Drawing for the job (mm, zero at the part's lowest x, y, z). A direction names the side the tool comes from. Give positions to 0.01 mm unless a question says otherwise; leave off trailing zeros. Loops run counter-clockwise (first coordinate to the right, second up) from the corner with the lowest first, then second, coordinate; pieces in that order, holes last. Notation, with made-up numbers: (56.25, 54) - (62.25, 54) arc R24 cw to (62.25, 69) - close; hole circle Ø7 at (-23.75, 55.5). An arc over 180 degrees is marked (long way). Return JSON: item names as keys, results as strings. Group by question number.
1) Drill centre lines: probe 1 along X at (y, z) = (75, 12.5); probe 2 along Z at (x, y) = (63.5, 78.5); probe 3 along X at (y, z) = (26.5, 34). Where is each one in solid material? Low to high. Write a range as from..to.
2) Mould opens along Z. For the marked faces 3, 4, 5 and 6 say: released by +Z, released by -Z, zero draft, split by the parting line, or undercut.
3) 3-axis set-ups, long thin cutter, end or side, ignore diameter. For the marked faces 1 and 2: which of +Z, -Z, +X, -X, +Y, -Y reach the whole face in a straight line?
4) Drop flat-ended pins along their axis: pin 1 (4 mm diameter, centred on x = 40, y = 16.5, fed in from +Z); pin 2 (1 mm diameter, centred on x = 49, z = 7.5, fed in from -Y). Give the stop position or say it passes through.
5) Slice it at D-D (z = 25.4). List the corners of the cut face in (x, y).
6) Slice it at B-B (y = 37). List the corners of the cut face in (x, z).
7) Slice it at A-A (x = 63.5). List the corners of the cut face in (y, z).
8) Slice it at C-C (z = 17). List the corners of the cut face in (x, y).
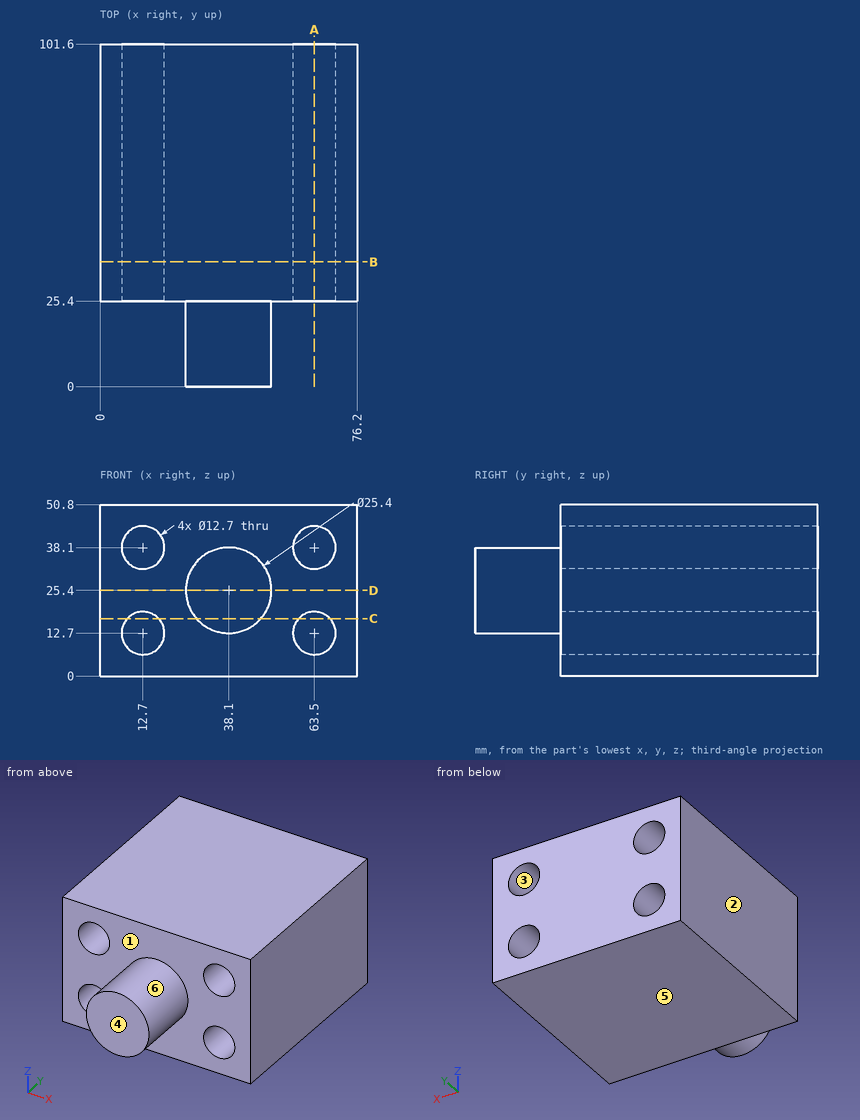
Results:
{
 "1": {"probe 1": "0..6.35, 19.05..57.15, 69.85..76.2", "probe 2": "0..6.35, 19.05..31.75, 44.45..50.8", "probe 3": "0..7.85, 17.55..58.65, 68.35..76.2"},
 "2": {"face 3": "undercut", "face 4": "zero draft", "face 5": "released by -Z", "face 6": "split by the parting line"},
 "3": {"face 1": "-Y", "face 2": "+Z, -Z, -X, +Y, -Y"},
 "4": {"pin 1": "z = 38.1", "pin 2": "y = 25.4"},
 "5": {"outline": "(0, 25.4) - (25.4, 25.4) - (25.4, 0) - (50.8, 0) - (50.8, 25.4) - (76.2, 25.4) - (76.2, 101.6) - (0, 101.6) - close"},
 "6": {"outline": "(0, 0) - (76.2, 0) - (76.2, 50.8) - (0, 50.8) - close; hole circle Ø12.7 at (12.7, 12.7); hole circle Ø12.7 at (12.7, 38.1); hole circle Ø12.7 at (63.5, 12.7); hole circle Ø12.7 at (63.5, 38.1)"},
 "7": {"outline": "(25.4, 0) - (101.6, 0) - (101.6, 6.35) - (25.4, 6.35) - close; (25.4, 19.05) - (101.6, 19.05) - (101.6, 31.75) - (25.4, 31.75) - close; (25.4, 44.45) - (101.6, 44.45) - (101.6, 50.8) - (25.4, 50.8) - close"},
 "8": {"outline": "(0, 25.4) - (8.03, 25.4) - (8.03, 101.6) - (0, 101.6) - close; (17.37, 25.4) - (28.57, 25.4) - (28.57, 0) - (47.63, 0) - (47.63, 25.4) - (58.83, 25.4) - (58.83, 101.6) - (17.37, 101.6) - close; (68.17, 25.4) - (76.2, 25.4) - (76.2, 101.6) - (68.17, 101.6) - close"}
}
